For this review, take the finished solid that the model builds, in its own axes (mm). Face numbers are marked on the shaded views. A direction names the side the tool comes from. Give positions to 0.01 mm unless a question says otherwise; leave off trailing zeros. Loops run counter-clockwise (first coordinate to the right, second up) from the corner with the lowest first, then second, coordinate; pieces in that order, holes last.
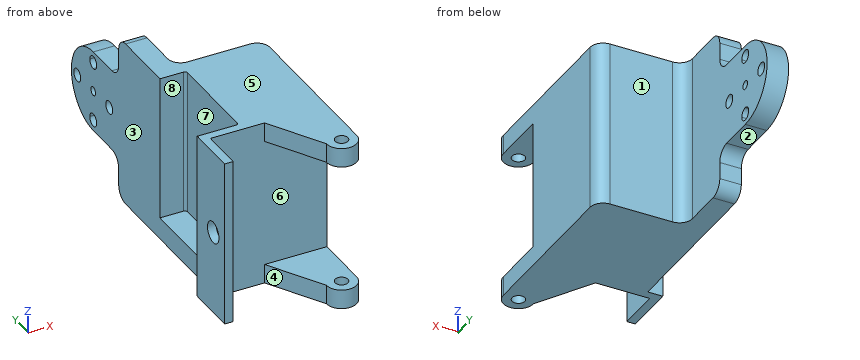
```python
from build123d import *

# Parameters (mm, degrees)
BOSS_EXTRUDE1_DEPTH      = 19.5
SKETCH3_W                = 2
SKETCH3_H                = 39
BOSS_EXTRUDE2_DEPTH      = 10
SKETCH4_R                = 2.5
CUT_EXTRUDE3_DEPTH       = 10
SKETCH5_W                = 5.1
SKETCH5_H                = 22.95
BOSS_EXTRUDE3_DEPTH      = 25.1
SKETCH8_W                = 15.5
SKETCH8_H                = 22.95
BOSS_EXTRUDE4_DEPTH      = 33.9
BOSS_EXTRUDE5_DEPTH      = 19.5
SKETCH12_W               = 30.263636296
SKETCH12_H               = 30
CUT_EXTRUDE6_DEPTH       = 16.5
SKETCH13_R               = 1.5
CUT_EXTRUDE7_DEPTH       = 64.966273157
FILLET3_R                = 3
SKETCH16_W               = 39
SKETCH16_H               = 3.05
BOSS_EXTRUDE6_DEPTH      = 25.1
SKETCH17_W               = 5
SKETCH17_H               = 39
BOSS_EXTRUDE7_DEPTH      = 15
FILLET4_R                = 3
FILLET11_R               = 0.6
FILLET12_R               = 0.6
SKETCH18_W               = 5
SKETCH18_H               = 19.16
BOSS_EXTRUDE12_DEPTH     = 25.725
CUT_EXTRUDE13_DEPTH      = 73.504038681
CUT_EXTRUDE13_DEPTH_BACK = 73.504038681
CUT_EXTRUDE14_DEPTH      = 73.504038681
FILLET15_R               = 3
FILLET16_R               = 3
FILLET17_R               = 3
FILLET18_R               = 3
SKETCH23_W               = 3.5
SKETCH23_H               = 39
CUT_EXTRUDE15_DEPTH      = 26


with BuildPart() as part:
    # Sketch1 → Boss-Extrude1 (new, symmetric)
    with BuildSketch(Plane.XY):
        Polygon((-18.427969187, 26), (-18.427969187, 0), (-43.527969187, 0), (-43.527969187, -2), (-14.427969187, -2), (-14.427969187, 26), align=None)
    extrude(amount=BOSS_EXTRUDE1_DEPTH, both=True)

    # Sketch3 → Boss-Extrude2 (add)
    with BuildSketch(Plane(origin=(0, -2, 0), x_dir=(1, 0, 0), z_dir=(0, 1, 0))):
        with Locations((-42.527969187, 0)):
            Rectangle(SKETCH3_W, SKETCH3_H)
    extrude(amount=-BOSS_EXTRUDE2_DEPTH)

    # Sketch4 → Cut-Extrude3 (cut)
    with BuildSketch(Plane(origin=(-41.527969187, 0, 0), x_dir=(0, 0, -1), z_dir=(1, 0, 0))):
        with Locations((0, -7)):
            Circle(SKETCH4_R)
    extrude(amount=-CUT_EXTRUDE3_DEPTH, mode=Mode.SUBTRACT)

    # Sketch5 → Boss-Extrude3 (add)
    with BuildSketch(Plane.ZY.offset(18.427969187)):
        with Locations((-16.95, 11.475)):
            Rectangle(SKETCH5_W, SKETCH5_H)
    extrude(amount=BOSS_EXTRUDE3_DEPTH)

    # Sketch8 → Boss-Extrude4 (add)
    with BuildSketch(Plane.XY.offset(-14.4)):
        with Locations((-26.177969187, 11.475)):
            Rectangle(SKETCH8_W, SKETCH8_H)
    extrude(amount=BOSS_EXTRUDE4_DEPTH)

    # Sketch11 → Boss-Extrude5 (add, symmetric)
    with BuildSketch(Plane.XY):
        with BuildLine():
            Line((-14.427969187, -2), (-14.427969187, -15))
            ThreePointArc((-14.427969187, -15), (-17.927969187, -18.5), (-21.427969187, -15))
            Line((-21.427969187, -15), (-28.933522687, -2))
            Line((-28.933522687, -2), (-14.427969187, -2))
        make_face()
    extrude(amount=BOSS_EXTRUDE5_DEPTH, both=True)

    # Sketch12 → Cut-Extrude6 (cut)
    with BuildSketch(Plane(origin=(0, -18.5, 0), x_dir=(1, 0, 0), z_dir=(0, 1, 0))):
        with Locations((-18.965310336, 0)):
            Rectangle(SKETCH12_W, SKETCH12_H)
    extrude(amount=CUT_EXTRUDE6_DEPTH, mode=Mode.SUBTRACT)

    # Sketch13 → Cut-Extrude7 (cut, through all)
    with BuildSketch(Plane.XY.offset(19.5)):
        with Locations((-17.927969187, -15)):
            Circle(SKETCH13_R)
    extrude(amount=-CUT_EXTRUDE7_DEPTH, mode=Mode.SUBTRACT)

    # Fillet3
    fillet3_edges = [part.edges().sort_by_distance(p)[0] for p in [
        (-14.427969187, 26, 0),
    ]]
    fillet(fillet3_edges, radius=FILLET3_R)

    # Sketch16 → Boss-Extrude6 (add)
    with BuildSketch(Plane.ZY.offset(18.427969187)):
        with Locations((0, 24.475)):
            Rectangle(SKETCH16_W, SKETCH16_H)
    extrude(amount=BOSS_EXTRUDE6_DEPTH)

    # Sketch17 → Boss-Extrude7 (add)
    with BuildSketch(Plane(origin=(0, 26, 0), x_dir=(1, 0, 0), z_dir=(0, 1, 0))):
        with Locations((-37.527969187, 0)):
            Rectangle(SKETCH17_W, SKETCH17_H)
    extrude(amount=BOSS_EXTRUDE7_DEPTH)

    # Fillet4
    fillet4_edges = [part.edges().sort_by_distance(p)[0] for p in [
        (-35.027969187, 26, 0),
    ]]
    fillet(fillet4_edges, radius=FILLET4_R)

    # Fillet11
    fillet11_edges = [part.edges().sort_by_distance(p)[0] for p in [
        (-33.927969187, 22.95, 2.55),
    ]]
    fillet(fillet11_edges, radius=FILLET11_R)

    # Fillet12
    fillet12_edges = [part.edges().sort_by_distance(p)[0] for p in [
        (-33.927969187, 0, 2.55),
    ]]
    fillet(fillet12_edges, radius=FILLET12_R)

    # Sketch18 → Boss-Extrude12 (add)
    with BuildSketch(Plane(origin=(0, 41, 0), x_dir=(1, 0, 0), z_dir=(0, 1, 0))):
        with Locations((-37.527969187, 0)):
            Rectangle(SKETCH18_W, SKETCH18_H)
    extrude(amount=BOSS_EXTRUDE12_DEPTH)

    # Sketch20 → Cut-Extrude13 (cut, two sides: drawn at the far end of the back side and taken through both)
    with BuildSketch(Plane(origin=(-35.027969187, 0, 0), x_dir=(0, 0, -1), z_dir=(1, 0, 0)).offset(-CUT_EXTRUDE13_DEPTH_BACK)):
        with BuildLine():
            ThreePointArc((0, 46.65), (-1.5, 45.15), (0, 43.65))
            ThreePointArc((0, 43.65), (1.5, 45.15), (0, 46.65))
        make_face()
        with BuildLine():
            ThreePointArc((-7, 53.65), (-8.5, 52.15), (-7, 50.65))
            ThreePointArc((-7, 50.65), (-5.939339828, 51.089339828), (-5.5, 52.15))
            ThreePointArc((-5.5, 52.15), (-5.939339828, 53.210660172), (-7, 53.65))
        make_face()
        with BuildLine():
            ThreePointArc((0, 60.65), (-1.5, 59.15), (0, 57.65))
            ThreePointArc((0, 57.65), (1.5, 59.15), (0, 60.65))
        make_face()
        with BuildLine():
            ThreePointArc((7, 53.65), (5.939959741, 53.211279722), (5.500001024, 52.151752864))
            ThreePointArc((5.500001024, 52.151752864), (5.938720278, 51.089959741), (7, 50.65))
            ThreePointArc((7, 50.65), (8.5, 52.15), (7, 53.65))
        make_face()
        with BuildLine():
            ThreePointArc((1, 52.15), (0, 53.15), (-1, 52.15))
            ThreePointArc((-1, 52.15), (0, 51.15), (1, 52.15))
        make_face()
    extrude(amount=CUT_EXTRUDE13_DEPTH + CUT_EXTRUDE13_DEPTH_BACK, mode=Mode.SUBTRACT)

    # Sketch21 → Cut-Extrude14 (cut, through all)
    with BuildSketch(Plane(origin=(-35.027969187, 0, 0), x_dir=(0, 0, -1), z_dir=(1, 0, 0))):
        with BuildLine():
            Line((-9.58, 66.725), (9.58, 66.725))
            Line((9.58, 66.725), (9.58, 52.15))
            ThreePointArc((9.58, 52.15), (0, 61.73), (-9.58, 52.15))
            Line((-9.58, 52.15), (-9.58, 66.725))
        make_face()
    extrude(amount=-CUT_EXTRUDE14_DEPTH, mode=Mode.SUBTRACT)

    # Fillet15
    fillet15_edges = [part.edges().sort_by_distance(p)[0] for p in [
        (-37.527969187, 41, 9.58),
    ]]
    fillet(fillet15_edges, radius=FILLET15_R)

    # Fillet16
    fillet16_edges = [part.edges().sort_by_distance(p)[0] for p in [
        (-37.527969187, 41, 19.5),
    ]]
    fillet(fillet16_edges, radius=FILLET16_R)

    # Fillet17
    fillet17_edges = [part.edges().sort_by_distance(p)[0] for p in [
        (-37.527969187, 41, -19.5),
    ]]
    fillet(fillet17_edges, radius=FILLET17_R)

    # Fillet18
    fillet18_edges = [part.edges().sort_by_distance(p)[0] for p in [
        (-37.527969187, 41, -9.58),
    ]]
    fillet(fillet18_edges, radius=FILLET18_R)

    # Sketch23 → Cut-Extrude15 (cut)
    with BuildSketch(Plane(origin=(0, 26, 0), x_dir=(1, 0, 0), z_dir=(0, 1, 0))):
        with Locations((-41.777969187, 0)):
            Rectangle(SKETCH23_W, SKETCH23_H)
    extrude(amount=-CUT_EXTRUDE15_DEPTH, mode=Mode.SUBTRACT)


solid = part.part
```
Q1. For pin 1 Ø5 at (x, z) = (-36, 15.5) entering from +Y; pin 2 Ø4 at (y, z) = (-7, 0) entering from +X; pin 3 Ø10 at (y, z) = (44, -4) entering from +X; pin 4 Ø4.5 at (x, z) = (-37, -14) entering from +Y, all flat-tipped, find the tip position at first contact; note any pin that passes through.
Answers:
pin 1: stops at y = 41
pin 2: passes through
pin 3: stops at x = -35.03
pin 4: stops at y = 41.12
Q2. Consider section A-A on z = 0. Count the separate pieces of the cut face and the enclosed holes in it, plus the area to 3 significant figures.
Answers:
separate pieces: 5
enclosed holes: 0
area: 733 mm2
Q3. Consider section D-D on y = 59.15. Give the boundary of the cut face in (x, z), plus the area to 3 significant figures.
Answers:
outline: (-40.03, -6.54) - (-35.03, -6.54) - (-35.03, -1.5) - (-40.03, -1.5) - close; (-40.03, 1.5) - (-35.03, 1.5) - (-35.03, 6.54) - (-40.03, 6.54) - close
area: 50.4 mm2
Q4. For probe 1 along Y at (x, z) = (-42.25, 0); probe 2 along Y at (x, z) = (-31.5, 15); probe 3 along Y at (x, z) = (-39.75, 10), list the stretches that pass through material, from the lowest coordinate up.
Answers:
probe 1: y = -12 to -9.5, -4.5 to 0
probe 2: y = -2 to 26
probe 3: y = -2 to 0, 22.95 to 42.47
Q5. Consider section C-C on y = -7. Give the boundary of the cut face in (x, z).
Answers:
outline: (-43.53, -19.5) - (-41.53, -19.5) - (-41.53, -2.5) - (-43.53, -2.5) - close; (-43.53, 2.5) - (-41.53, 2.5) - (-41.53, 19.5) - (-43.53, 19.5) - close; (-26.05, -19.5) - (-14.43, -19.5) - (-14.43, -15) - (-26.05, -15) - close; (-26.05, 15) - (-14.43, 15) - (-14.43, 19.5) - (-26.05, 19.5) - close
Q6. Machinability: for the marked faces 1, 2, 3 and 4, which of the approach directions +Z, -Z, +X, -X, +Y, -Y give a long, thin tool a straight path to every point of the face, cutting with its end or side? Answer none if there is none.
Answers:
face 1: +Z, -Z, +X, +Y
face 2: -Z, +X, -X, +Y
face 3: +Z, -Z, -X, +Y
face 4: +Z, -Z, -Y
Q7. Consider section B-B on x = -37. Give the boundary of the cut face in (y, z).
Answers:
outline: (-2, -19.5) - (38, -19.5) arc R3 ccw to (41, -16.5) - (41, -12.58) arc R3 cw to (44, -9.58) - (52.15, -9.58) arc R9.58 ccw to (52.15, 9.58) - (44, 9.58) arc R3 cw to (41, 12.58) - (41, 16.5) arc R3 ccw to (38, 19.5) - (22.95, 19.5) - (22.95, -14.4) - (0, -14.4) - (0, 19.5) - (-2, 19.5) - close; hole circle Ø3 at (45.15, 0); hole circle Ø3 at (52.15, -7); hole circle Ø3 at (52.15, 7); hole circle Ø2 at (52.15, 0); hole circle Ø3 at (59.15, 0)
Q8. Mouldability with a two-part tool opening along Y and no side actions: class the marked faces 5, 6, 7 and 8 as +Y half, -Y half, draft (parallel to the pull), parting line (faces both ways), or undercut.
Answers:
face 5: draft
face 6: -Y half
face 7: undercut
face 8: undercut
